Verification items for the finished model (mm, model axes). A direction names the side the tool comes from. Coordinates: 2 decimals unless noted, no trailing zeros. Order: outer loops, then holes, each group sorted by start corner. A loop starts at its lowest first (then second) coordinate and runs counter-clockwise, first axis right, second up. Notation, with made-up numbers: M 20.5,-34 L 66.5,-34 A22 cw 66.5,-15 Z; hole C 42,2 d10. An arc over 180 degrees is marked long. Return JSON: item names as keys, results as strings. Group by question number.
1. Section check C-C, the plane x = -6.5. Record the cut outline in (y, z).
2. Section check B-B, the plane z = -8.5. Record the cut outline in (x, y), plus the area to 3 significant figures.
3. Material ranges on line 1 along X through (y, z) = (-4.25, -20); line 2 along Z through (x, y) = (3.5, -18.25); line 3 along Y through (x, z) = (-6.5, -10), recorded low to high.
4. Set-up check for faces 4 (the cylindrical face through (35.301, -11.619, 22.272)), 5 (the flat face through (8, -11, -28.873)): record each of +Z, -Z, +X, -X, +Y, -Y from which the full face is reachable in a straight line by a thin tool's end or side.
5. Section check A-A, the plane y = -6.5. Record the cut outline in (x, z).
6. Mould release check, pull along X, two halves, no side actions. Record for faces 1 (the flat face through (8, -11, -30.873)), 2 (the flat face through (8, -2, -4)), 3 (the cylindrical face through (-18.941, -11.619, 22.225)): +X half, -X half, draft (parallel to the pull), parting line (faces both ways), or undercut.
```python
from build123d import *

# Parameters (mm, degrees)
F0_W     = 56
F0_H     = 54
F1_DEPTH = 20
F3_DEPTH = 18
F4_R     = 3
F5_R     = 3


with BuildPart() as f1:
    # F0 (on Front) → F1 (new body)
    with BuildSketch(Plane.XZ):
        with Locations((8.203572, -3.872868)):
            Rectangle(F0_W, F0_H)
    extrude(amount=F1_DEPTH)

    # F2 (on face) → F3 (cut)
    with BuildSketch(Plane.XZ.offset(20)):
        with BuildLine():
            Line((29.203572, 21.127132), (-12.796428, 21.127132))
            ThreePointArc((-12.796428, 21.127132), (-16.331962, 19.662666), (-17.796428, 16.127132))
            Line((-17.796428, 16.127132), (-17.796428, -23.872868))
            ThreePointArc((-17.796428, -23.872868), (-16.331962, -27.408402), (-12.796428, -28.872868))
            Line((-12.796428, -28.872868), (29.203572, -28.872868))
            ThreePointArc((29.203572, -28.872868), (32.739106, -27.408402), (34.203572, -23.872868))
            Line((34.203572, -23.872868), (34.203572, 16.127132))
            ThreePointArc((34.203572, 16.127132), (32.739106, 19.662666), (29.203572, 21.127132))
        make_face()
    extrude(amount=-F3_DEPTH, mode=Mode.SUBTRACT)

    # F4
    f4_edges = [f1.edges().sort_by_distance(p)[0] for p in [
        (36.203572, -10, 23.127132),
        (-19.796428, -10, 23.127132),
        (36.203572, -10, -30.872868),
        (-19.796428, -10, -30.872868),
    ]]
    fillet(f4_edges, radius=F4_R)

    # F5
    f5_edges = [f1.edges().sort_by_distance(p)[0] for p in [
        (8.203572, 0, 23.127132),
    ]]
    fillet(f5_edges, radius=F5_R)


solid = f1.part
```
Answers follow:
{
 "1": {"outline": "M -20,-30.87 L -3,-30.87 A3 ccw 0,-27.87 L 0,20.13 A3 ccw -3,23.13 L -20,23.13 L -20,21.13 L -2,21.13 L -2,-28.87 L -20,-28.87 Z"},
 "2": {"outline": "M -19.8,-20 L -17.8,-20 L -17.8,-2 L 34.2,-2 L 34.2,-20 L 36.2,-20 L 36.2,-3 A3 ccw 33.2,0 L -16.8,0 A3 ccw -19.8,-3 Z", "area": "180 mm^2"},
 "3": {"line 1": "-19.8 to -17.8, 34.2 to 36.2", "line 2": "-30.87 to -28.87, 21.13 to 23.13", "line 3": "-2 to 0"},
 "4": {"face 4": "+Z, +X, +Y, -Y", "face 5": "-Y"},
 "5": {"outline": "M -19.8,-27.87 A3 ccw -16.8,-30.87 L 33.2,-30.87 A3 ccw 36.2,-27.87 L 36.2,20.13 A3 ccw 33.2,23.13 L -16.8,23.13 A3 ccw -19.8,20.13 Z; hole M -17.8,-23.87 A5 ccw -12.8,-28.87 L 29.2,-28.87 A5 ccw 34.2,-23.87 L 34.2,16.13 A5 ccw 29.2,21.13 L -12.8,21.13 A5 ccw -17.8,16.13 Z"},
 "6": {"face 1": "draft", "face 2": "undercut", "face 3": "-X half"}
}
